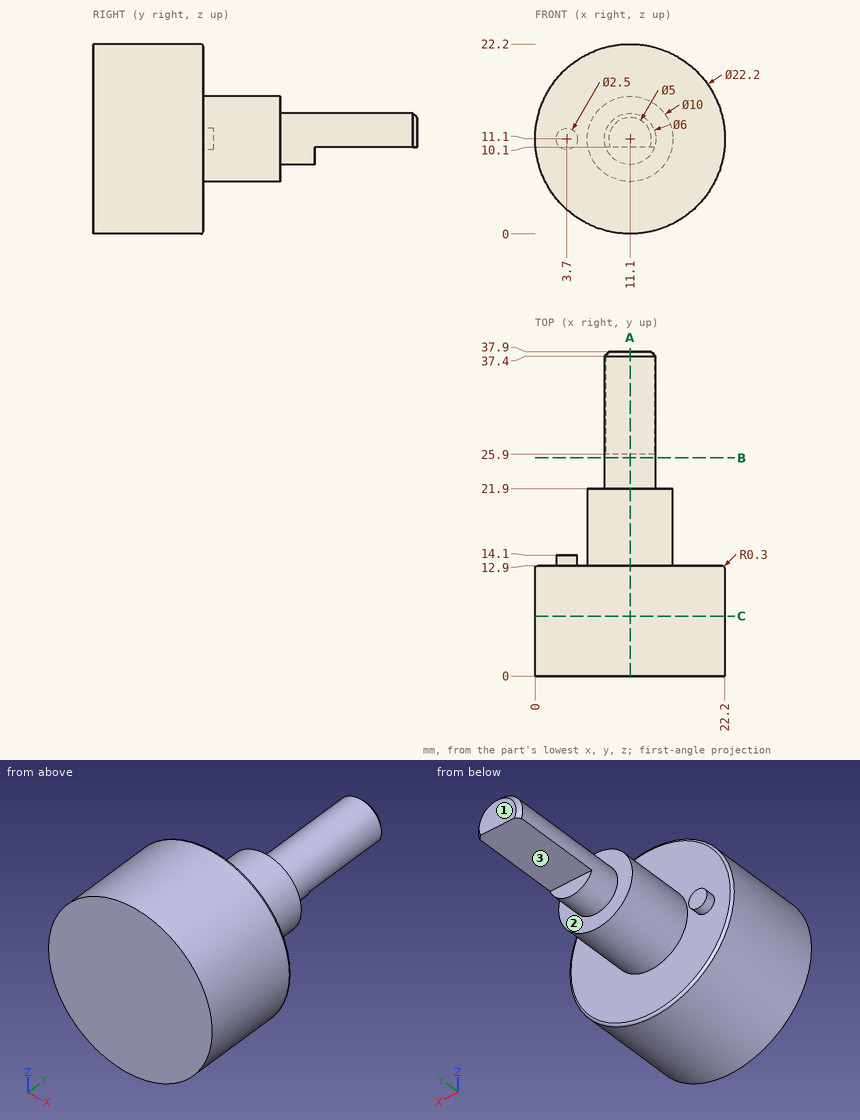
Geometry: see drawing. Coordinates: mm, zero at the bounding-box minimum. A direction names the side the tool comes from. Coordinates: 2 decimals unless noted, no trailing zeros. Order: outer loops, then holes, each group sorted by start corner. A loop starts at its lowest first (then second) coordinate and runs counter-clockwise, first axis right, second up. Notation, with made-up numbers: (7.5, 72.5) - (19.5, 72.5) arc R30 ccw to (19.5, 106.5) - close; hole circle Ø9 at (-11, 76). An arc over 180 degrees is marked (long way). Use one line per item in the form item = value.
1) Pin query (flat end, axial travel): pin 1 (0.6 mm diameter, centred on x = 12, z = 9, fed in from +Y); pin 2 (6 mm diameter, centred on x = 12, y = 33, fed in from -Z); pin 3 (1.2 mm diameter, centred on x = 3, z = 11, fed in from +Y); pin 4 (1.5 mm diameter, centred on y = 34, z = 16, fed in from +X). Return the tip coordinate at first contact, or that it passes through.
Solutions:
pin_1 = 25.9
pin_2 = 10.1
pin_3 = 14.1
pin_4 = through
2) Section B-B (y = 25.5). Return loops of the section in (x, z), then the cut area to 3 significant figures.
Solutions:
outline = circle Ø6 at (11.1, 11.1)
area = 28.3 mm^2
3) Set-up query: the marked faces 1, 2 and 3. Return all of +Z, -Z, +X, -X, +Y, -Y with unobstructed straight access to the full face (end or side cutting, diameter ignored); none if empty.
Solutions:
face_1 = +Z, -Z, +X, -X, +Y
face_2 = +Y
face_3 = -Z, +X, -X, +Y
4) Section A-A (x = 11.1). Return loops of the section in (y, z), then the cut area to 3 significant figures.
Solutions:
outline = (0, 0) - (12.6, 0) arc R0.3 ccw to (12.9, 0.3) - (12.9, 6.1) - (21.9, 6.1) - (21.9, 8.1) - (25.9, 8.1) - (25.9, 10.1) - (37.9, 10.1) - (37.9, 13.6) - (37.4, 14.1) - (21.9, 14.1) - (21.9, 16.1) - (12.9, 16.1) - (12.9, 21.9) arc R0.3 ccw to (12.6, 22.2) - (0, 22.2) - close
area = 448 mm^2
5) Section C-C (y = 7). Return loops of the section in (x, z), then the cut area to 3 significant figures.
Solutions:
outline = circle Ø22.2 at (11.1, 11.1)
area = 387 mm^2
6) Ray query, L1, parallel to Y at x = 5, z = 15; L2, parallel to Y at x = 6.5, z = 11.5; L3, parallel to X at y = 15.5, z = 9.75. Return the intervals inside material, ascending.
Solutions:
L1 = 0 to 12.9
L2 = 0 to 21.9
L3 = 6.29 to 15.91
